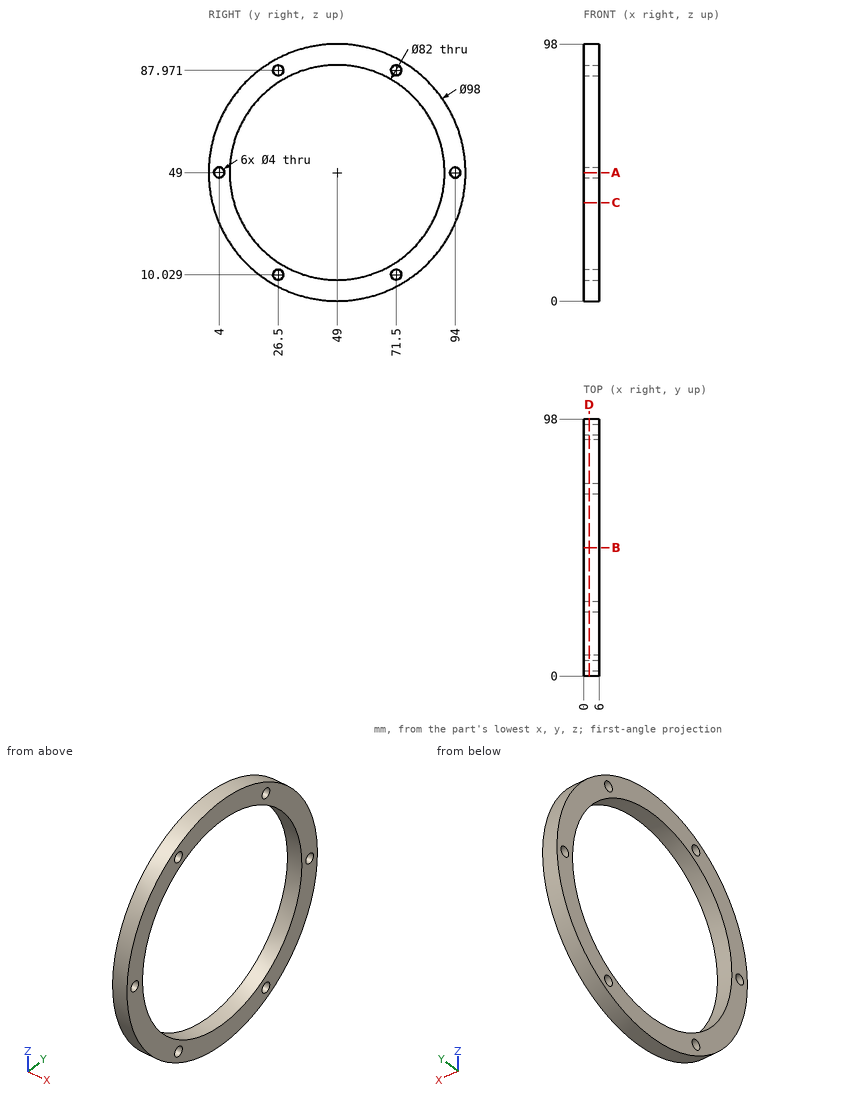
Design review of the part shown in the three views and the two pictorial views. Dimensions are in mm from the part's minimum x, y and z. Give positions to 0.01 mm unless a question says otherwise; leave off trailing zeros. Write each loop counter-clockwise with the first axis right and the second up, starting at its lowest first coordinate (ties: lowest second). Pieces come first, ordered by that corner, then holes. Notation, with made-up numbers: M 12.25,12 L 68.25,12 A14 ccw 68.25,28 Z; hole C -26,87 d1. An arc over 180 degrees is marked long. One line per question, with ' | ' between items. Start each with the question number.
Item 1: We need section A-A on z = 49. Write out the cut boundary in (x, y), plus the area to 3 significant figures.
Item 2: Wall thickness on line 1 (Y direction, x = 1.35, z = 49); line 2 (Z direction, x = 1.3, y = 64); line 3 (Y direction, x = 3.8, z = 18): over which ranges is each line inside the solid? List them lowest first. Write a range as from..to.
Item 3: For pin 1 (2.5 mm diameter, centred on y = 71.5, z = 87.97, fed in from +X); pin 2 (1 mm diameter, centred on x = 4, z = 38, fed in from +Y); pin 3 (3 mm diameter, centred on x = 4, y = 57.5, fed in from -Z), all flat-tipped, find the tip position at first contact; note any pin that passes through.
Item 4: We need section C-C on z = 37.5. Write out the cut boundary in (x, y), plus the area to 3 significant figures.
Item 5: We need section D-D on x = 2.1. Write out the cut boundary in (y, z), plus the area to 3 significant figures.
Item 6: We need section B-B on y = 49. Write out the cut boundary in (x, z), plus the area to 3 significant figures.
Results found:
1) outline: M 0,0 L 6,0 L 6,2 L 0,2 Z; M 0,6 L 6,6 L 6,8 L 0,8 Z; M 0,90 L 6,90 L 6,92 L 0,92 Z; M 0,96 L 6,96 L 6,98 L 0,98 Z | area: 48.0 mm2
2) line 1: y = 0..2, 6..8, 90..92, 96..98 | line 2: z = 2.35..10.84, 87.16..95.65 | line 3: y = 11.05..22.17, 75.83..86.95
3) pin 1: passes through | pin 2: stops at y = 96.86 | pin 3: stops at z = 0.5
4) outline: M 0,1.37 L 6,1.37 L 6,9.65 L 0,9.65 Z; M 0,88.35 L 6,88.35 L 6,96.63 L 0,96.63 Z | area: 99.3 mm2
5) outline: C 49,49 d98; hole C 4,49 d4; hole C 49,49 d82; hole C 26.5,10.03 d4; hole C 26.5,87.97 d4; hole C 71.5,10.03 d4; hole C 71.5,87.97 d4; hole C 94,49 d4 | area: 2,190 mm2
6) outline: M 0,0 L 6,0 L 6,8 L 0,8 Z; M 0,90 L 6,90 L 6,98 L 0,98 Z | area: 96.0 mm2
